Build history of the part. All positions in model axes, mm. A direction names the side the tool comes from. Coordinates: 2 decimals unless noted, no trailing zeros. Write each loop counter-clockwise with the first axis right and the second up, starting at its lowest first coordinate (ties: lowest second). Pieces come first, ordered by that corner, then holes.
from build123d import *

# Parameters (mm, degrees)
F0_W     = 28
F0_H     = 60
F3_R     = 30
F3_R_2   = 7
F4_DEPTH = 7
F5_COUNT = 5


with BuildPart() as f1:
    # F0 (on Front) → F1 (revolve)
    with BuildSketch(Plane.XZ):
        Polygon((-52, 78), (0, 78), (0, 80), (-28, 80), (-52, 80), align=None)
        with Locations((-14, 110)):
            Rectangle(F0_W, F0_H)
        Polygon((-52, 0), (-52, 78), (-52, 80), (-58, 80), (-58, 0), align=None)
    revolve(axis=Axis((-29, 0, 0), (1, 0, 0)))

    # F3 (on offset) → F4 (cut)
    with BuildSketch(Plane.YZ.offset(-58)):
        Circle(F3_R)
        with Locations((0, 57)):
            Circle(F3_R_2)
    f4 = extrude(amount=F4_DEPTH, mode=Mode.SUBTRACT)

    # F5: F4 ×5 about axis
    f5_axis = Axis((-58, 0, 0), (1, 0, 0))
    for i in range(1, F5_COUNT):
        add(f4.solids().sort_by_distance((-54.5, -7, 57))[0].rotate(f5_axis, i * 360 / F5_COUNT), mode=Mode.SUBTRACT)


solid = f1.part
(1) 3-axis set-ups, long thin cutter, end or side, ignore diameter. For faces 5 (the cylindrical face through (-25.636, -77.336, -10.154)), 6 (the cylindrical face through (-55.04, -0.91, 63.94)), 7 (the flat face through (-28, 60, -60)): which of +Z, -Z, +X, -X, +Y, -Y reach the whole face in a straight line?
(2) Two-plate mould, pull along Z, no slides. Class faces 1 (the flat face through (-58, 34, -1)), 2 (the cylindrical face through (-55.04, 47.24, 16.95)), 3 (the cylindrical face through (-55, 30.7, -39.7)), 4 (the cylindrical face through (-43.21, 78.1, -17.34)): pulls with the +Z half, pulls with the -Z half, needs draft (parallel to the pull), parting line crosses it, or undercut.
(3) Slice it at A-A, the plane z = 0. List the corners of the cut face in (x, y).
(4) Probe L1, parallel to Z at x = -55.7, y = 0; L2, parallel to X at y = -94, z = 45.5; L3, parallel to X at y = 22, z = -42.5. List the from-to ranges inside material, lowest first.
(5) Slice it at B-B, the plane y = 0. List the corners of the cut face in (x, z).
(6) Slice it at C-C, the plane x = -4. List the corners of the cut face in (y, z), and give its area (3 significant figures).
(7) Slice it at D-D, the plane z = 70.5. List the corners of the cut face in (x, y).
(8) Flat gauge pins, fed straight in: P1, Ø1.5, axis at y = 38, z = -80, coming from the -X side; P2, Ø2, axis at x = -36.5, z = 70.5, coming from the -Y side; P3, Ø2, axis at x = -35, y = 11.5, coming from the +Z side. Where does each tip first touch, or does it go through?
Results:
1. face 5: +X
1. face 6: +X, -X
1. face 7: -X
2. face 1: needs draft
2. face 2: undercut
2. face 3: undercut
2. face 4: parting line crosses it
3. outline: (-58, -80) - (-28, -80) - (-28, -140) - (0, -140) - (0, -78) - (-52, -78) - (-52, -30) - (-58, -30) - close; (-58, 30) - (-52, 30) - (-52, 78) - (0, 78) - (0, 140) - (-28, 140) - (-28, 80) - (-58, 80) - close
4. L1: z = -80 to -30, 30 to 50, 64 to 80
4. L2: x = -28 to 0
4. L3: x = -58 to -52
5. outline: (-58, -80) - (-28, -80) - (-28, -140) - (0, -140) - (0, -78) - (-52, -78) - (-52, -30) - (-58, -30) - close; (-58, 30) - (-52, 30) - (-52, 50) - (-58, 50) - close; (-58, 64) - (-52, 64) - (-52, 78) - (0, 78) - (0, 140) - (-28, 140) - (-28, 80) - (-58, 80) - close
6. outline: circle Ø280 at (0, 0); hole circle Ø156 at (0, 0)
6. area: 42,500 mm2
7. outline: (-58, -37.81) - (-28, -37.81) - (-28, -120.95) - (0, -120.95) - (0, -33.37) - (-52, -33.37) - (-52, 33.37) - (0, 33.37) - (0, 120.95) - (-28, 120.95) - (-28, 37.81) - (-58, 37.81) - close
8. P1: stops at x = -28
8. P2: stops at y = -39.62
8. P3: stops at z = 79.31
